Autodesk Inventor part; units mm, degrees
ref_plane "YZ Plane" through (0, 0, 0) normal (1, 0, 0) x (0, 1, 0)
ref_plane "XZ Plane" through (0, 0, 0) normal (0, 1, 0) x (-1, 0, 0)
ref_plane "XY Plane" through (0, 0, 0) normal (0, 0, 1) x (1, 0, 0)
sketch "Sketch1" plane through (0, 0, 0) normal (0, 1, 0) x (-1, 0, 0)
  line L0 (-50, 50) -> (50, 50)
  line L1 (50, 50) -> (50, -50)
  line L2 (50, -50) -> (-50, -50)
  line L3 (-50, -50) -> (-50, 50)
  line L4 (-50, 50) -> (50, -50) construction
  line L5 (50, 50) -> (-50, -50) construction
  point P0 (0, 0)
  dimension "d0" = 100
  dimension "d1" = 100
extrude "Extrusion1" add sketch "Sketch1" along normal blind 100
sketch "Sketch2" plane through (0, 100, 0) normal (0, 1, 0) x (1, 0, 0)
  line L0 (50, 50) -> (-50, 50)
  line L1 (-50, 50) -> (-50, -50)
  line L2 (-50, -50) -> (50, -50)
  line L3 (50, -50) -> (50, 50)
  line L4 (50, -50) -> (-50, 50)
  line L5 (-50, 50) -> (-50, -50)
  line L6 (-50, -50) -> (50, 50)
  circle A0 centre (0, 0) radius 2.5
  dimension "d4" = 5
extrude "Extrusion2" add sketch "Sketch2" along normal blind 13 contours A0 L4 L6 | L6 L4 A0 | L4 L6 A0 | A0 L6 L4
sketch "Sketch3" plane through (50, 0, 50) normal (1, 0, 0) x (0, 0, -1)
  line L0 (0, 0) -> (100, 0)
  line L1 (100, 0) -> (100, 100)
  line L2 (0, 100) -> (100, 100)
  line L3 (0, 0) -> (0, 100)
  line L4 (96, 96) -> (96, 4)
  line L5 (96, 4) -> (4, 4)
  line L6 (4, 4) -> (4, 96)
  line L7 (4, 96) -> (96, 96)
  point P0 (50, 0)
  dimension "d7" = 4
extrude "Extrusion3" cut sketch "Sketch3" against normal blind 1 contours L4 L5 L6 L7
sketch "Sketch4" plane through (0, 100, 0) normal (0, 1, 0) x (1, 0, 0)
  circle A0 centre (0, 0) radius 2.5
  circle A1 centre (0, 0) radius 49
  circle A2 centre (0, 0) radius 14.7708
  line L0 (50, -50) -> (50, 50)
  line L1 (0, 0) -> (50, 50)
  line L2 (-50, -50) -> (50, -50)
  line L3 (0, 0) -> (50, -50)
  line L4 (0, -50) -> (0, 50)
  line L5 (50, 50) -> (-50, 50)
  line L6 (-1, -50) -> (-1, 50)
  line L7 (50.7071, -49.2929) -> (1.4142, 0)
  line L8 (1.4142, 0) -> (50.7071, 49.2929)
  line L9 (49.2929, -50.7071) -> (-1.4142, 0)
  line L10 (-1.4142, 0) -> (49.2929, 50.7071)
  line L11 (0, 0) -> (50, 0)
  line L12 (0, -1) -> (50, -1)
  line L13 (0, 1) -> (50, 1)
  point P0 (9.7134, 11.1276)
  point P1 (33.9339, 35.3481)
  point P2 (0, 49)
  point P3 (0, 14.7708)
  point P4 (14.7369, 1)
  point P5 (48.9898, 1)
  point P6 (35.3481, 33.9339)
  point P7 (11.1276, 9.7134)
  point P8 (33.9339, -35.3481)
  point P9 (9.7134, -11.1276)
  point P10 (0, -14.7708)
  point P11 (0, -49)
  point P12 (48.9898, -1)
  point P13 (14.7369, -1)
  point P14 (11.1276, -9.7134)
  point P15 (35.3481, -33.9339)
  dimension "d10" = 1
  dimension "d11" = 1
  dimension "d12" = 1
  dimension "d13" = 1
  dimension "d14" = 1
extrude "Extrusion4" cut sketch "Sketch4" against normal blind 1 contours A2 L8 A1 L13 | L12 A1 L7 A2 | A2 L4 A1 L10 | L9 A1 L4 A2
properties part number "stepper_box"
For this review, take the finished solid that the model builds, in its own axes (mm). A direction names the side the tool comes from. Give positions to 0.01 mm unless a question says otherwise; leave off trailing zeros. Loops run counter-clockwise (first coordinate to the right, second up) from the corner with the lowest first, then second, coordinate; pieces in that order, holes last. Notation, with made-up numbers: M -5.75,6 L 28.25,6 A8 cw 28.25,16 Z; hole C 89.5,-24.75 d8. An arc over 180 degrees is marked long. One line per item, written item: value. Start each with the question number.
Q1. Clearance check with flat-ended pins moving along their axes: pin 1 Ø10 at (x, z) = (38.5, -17) entering from +Y; pin 2 Ø10 at (x, y) = (-34.5, 101.5) entering from +Z; pin 3 Ø2 at (y, z) = (13, 15) entering from +X; pin 4 Ø0.8 at (x, z) = (49.5, 1.5) entering from +Y. State where each tip first meets the part, or that it passes through.
Q2. Machinability: for faces 1 (the face through (34, 99, 14)), 2 (the face through (-1, 49, -50)), 3 (the face through (49, 51, 1)), which of the approach directions +Z, -Z, +X, -X, +Y, -Y give a long, thin tool a straight path to every point of the face, cutting with its end or side? Answer none if there is none.
Q3. Add section B-B (x = -43). Give the boundary of the cut face in (y, z), and give its area (3 significant figures).
Q4. Add section A-A (z = -17.5). Give the boundary of the cut face in (x, y), and give its area (3 significant figures).
Q5. For L1, parallel to Y at x = -12, z = -35.5; L2, parallel to X at y = 62, z = -5.5; L3, parallel to Y at x = 13, z = -37, list the stretches that pass through material, from the lowest coordinate up.
Q6. Draft analysis for pull direction X (two halves, no side actions). For faces 4 (the face through (-50, 49, 1)), 5 (the face through (1, 49, 50)), 6 (the face through (13.672, 99.507, -5.59)), 7 (the face through (45.17, 99.51, 18.99)), state which applies: released by +X, released by -X, zero draft, split by the parting line, or undercut.
Reply:
1. pin 1: y = 99
1. pin 2: z = 50
1. pin 3: x = 49
1. pin 4: y = 100
2. face 1: +Y
2. face 2: -Z, +X, -X, +Y, -Y
2. face 3: +X
3. outline: M 0,-50 L 100,-50 L 100,50 L 0,50 Z
3. area: 10,000 mm²
4. outline: M -50,0 L 50,0 L 50,4 L 49,4 L 49,96 L 50,96 L 50,100 L 45.77,100 L 45.77,99 L 18.91,99 L 18.91,100 L 16.09,100 L 16.09,99 L 0,99 L 0,100 L -50,100 Z
4. area: 9,870 mm²
5. L1: 0 to 100
5. L2: -50 to 49
5. L3: 0 to 99
6. face 4: released by -X
6. face 5: zero draft
6. face 6: undercut
6. face 7: undercut
